```python
from build123d import *

# Parameters (mm, degrees)
SKETCH1_R           = 22.5
BOSS_EXTRUDE1_DEPTH = 5
SKETCH2_R           = 15
SKETCH2_R_2         = 12.1
BOSS_EXTRUDE2_DEPTH = 45
SKETCH3_R           = 2
CUT_EXTRUDE1_DEPTH  = 5


with BuildPart() as part:
    # Sketch1 → Boss-Extrude1 (new body)
    with BuildSketch(Plane.XY):
        Circle(SKETCH1_R)
    extrude(amount=BOSS_EXTRUDE1_DEPTH)

    # Sketch2 → Boss-Extrude2 (add)
    with BuildSketch(Plane.XY.offset(5)):
        Circle(SKETCH2_R)
        Circle(SKETCH2_R_2, mode=Mode.SUBTRACT)
    extrude(amount=BOSS_EXTRUDE2_DEPTH)

    # Sketch3 → Cut-Extrude1 (cut)
    with BuildSketch(Plane.XY.offset(5)):
        with Locations((0, 18.75)):
            Circle(SKETCH3_R)
        with Locations((16.237976321, 9.375)):
            Circle(SKETCH3_R)
        with Locations((16.237976321, -9.375)):
            Circle(SKETCH3_R)
        with Locations((0, -18.75)):
            Circle(SKETCH3_R)
        with Locations((-16.237976321, -9.375)):
            Circle(SKETCH3_R)
        with Locations((-16.237976321, 9.375)):
            Circle(SKETCH3_R)
    extrude(amount=-CUT_EXTRUDE1_DEPTH, mode=Mode.SUBTRACT)


solid = part.part
```
Geometry: final body of the model. Coordinates: model frame, mm. A direction names the side the tool comes from. Round coordinates to 2 decimals unless told otherwise and drop trailing zeros. Loops run counter-clockwise (first coordinate to the right, second up) from the corner with the lowest first, then second, coordinate; pieces in that order, holes last. Notation, with made-up numbers: (-30.75, 15.25) -> (-20.75, 15.25) arc R21 ccw to (-20.75, 46.25) -> close; hole circle Ø3 at (47, 82). An arc over 180 degrees is marked (long way). Use one line per item in the form item = value. Start each with the question number.
1) Line query: L1, parallel to Y at x = 0, z = 1.75; L2, parallel to Y at x = 0, z = 39.5; L3, parallel to X at y = -18, z = 1. Output: solid intervals per line, ascending.
2) Section C-C on y = 18.75. Output: boundary loops of the cut face in (x, z).
3) First-contact query: P1, Ø10, axis at x = -0.5, z = 25.5, coming from the +Y side; P2, Ø5, axis at x = -16.24, y = -9.38, coming from the +Z side; P3, Ø8, axis at y = -6.5, z = 7.5, coming from the -X side. Flat tips, straight axial feed; report the tip coordinate or a pass-through.
4) Section A-A on x = 0. Output: boundary loops of the cut face in (y, z).
5) Section B-B on y = -8.5. Output: boundary loops of the cut face in (x, z).
6) Draft query along X for faces 3 (the cylindrical face through (10.382, -19.961, 2.465)), 4 (the cylindrical face through (17.313, 11.061, 2.535)), 5 (the flat face through (1, 12.3, 50)), 6 (the flat face through (0, 0, 5)). Return one class per face: released by +X, released by -X, zero draft, split by the parting line, or undercut.
7) Access query for faces 1 (the flat face through (0, 0, 0)), 2 (the cylindrical face through (11.18, -4.63, 27.18)). Directions: +Z, -Z, +X, -X, +Y, -Y. A direction counts if a zero-diameter tool reaches every point of the face in a straight line with its end or side. Return the directions, or none.
8) Section D-D on z = 10. Output: boundary loops of the cut face in (x, y).
Response:
q1.L1 = -22.5 to -20.75, -16.75 to 16.75, 20.75 to 22.5
q1.L2 = -15 to -12.1, 12.1 to 15
q1.L3 = -13.5 to -1.85, 1.85 to 13.5
q2.outline = (-12.44, 0) -> (-2, 0) -> (-2, 5) -> (-12.44, 5) -> close; (2, 0) -> (12.44, 0) -> (12.44, 5) -> (2, 5) -> close
q3.P1 = 15
q3.P2 = 5
q3.P3 = -22.25
q4.outline = (-22.5, 0) -> (-20.75, 0) -> (-20.75, 5) -> (-22.5, 5) -> close; (-16.75, 0) -> (16.75, 0) -> (16.75, 5) -> (15, 5) -> (15, 50) -> (12.1, 50) -> (12.1, 5) -> (-12.1, 5) -> (-12.1, 50) -> (-15, 50) -> (-15, 5) -> (-16.75, 5) -> close; (20.75, 0) -> (22.5, 0) -> (22.5, 5) -> (20.75, 5) -> close
q5.outline = (-20.83, 0) -> (-18.04, 0) -> (-18.04, 5) -> (-20.83, 5) -> close; (-14.44, 0) -> (14.44, 0) -> (14.44, 5) -> (12.36, 5) -> (12.36, 50) -> (8.61, 50) -> (8.61, 5) -> (-8.61, 5) -> (-8.61, 50) -> (-12.36, 50) -> (-12.36, 5) -> (-14.44, 5) -> close; (18.04, 0) -> (20.83, 0) -> (20.83, 5) -> (18.04, 5) -> close
q6.face_3 = split by the parting line
q6.face_4 = undercut
q6.face_5 = zero draft
q6.face_6 = undercut
q7.face_1 = -Z, +X, -X, +Y, -Y
q7.face_2 = +Z
q8.outline = circle Ø30 at (0, 0); hole circle Ø24.2 at (0, 0)
